Build history of the part. All positions in model axes, mm. Face numbers are marked on the shaded views. A direction names the side the tool comes from. Give positions to 0.01 mm unless a question says otherwise; leave off trailing zeros. Order: outer loops, then holes, each group sorted by start corner. A loop starts at its lowest first (then second) coordinate and runs counter-clockwise, first axis right, second up. Notation, with made-up numbers: M 26,-26.5 L 83,-26.5 A18 ccw 83,0.5 Z; hole C 83,44.25 d3. An arc over 180 degrees is marked long. One line per item, written item: value. Start each with the question number.
from build123d import *

# Parameters (mm, degrees)
SKICA1_W                 = 50
SKICA1_H                 = 65
P_IDAT_VYSUNUT_M1_DEPTH  = 30
P_IDAT_VYSUNUT_M2_DEPTH  = 50
ODEBRAT_VYSUNUT_M1_DEPTH = 18.9
SKICA6_R                 = 2.8
ODEBRAT_VYSUNUT_M2_DEPTH = 58.744783314
SKICA7_R                 = 7.5
ODEBRAT_VYSUNUT_M3_DEPTH = 8.7
SKICA8_R                 = 2.35
ODEBRAT_VYSUNUT_M4_DEPTH = 8.5


with BuildPart() as part:
    # Skica1 → Přidat vysunutím1 (new body)
    with BuildSketch(Plane.XY):
        Rectangle(SKICA1_W, SKICA1_H)
    extrude(amount=P_IDAT_VYSUNUT_M1_DEPTH)

    # Skica3 → Přidat vysunutím2 (add, through all)
    with BuildSketch(Plane(origin=(25, 0, 0), x_dir=(0, 0, -1), z_dir=(1, 0, 0))):
        Polygon((0, 32.5), (0, 48.5), (-30, 32.5), align=None)
    extrude(amount=-P_IDAT_VYSUNUT_M2_DEPTH)

    # Skica5 → Odebrat vysunutím1 (cut)
    with BuildSketch(Plane.XY.offset(30)):
        Polygon((-20.3, 31.35), (20.31, 31.35), (22.6, -31.35), (-22.6, -31.35), align=None)
    extrude(amount=-ODEBRAT_VYSUNUT_M1_DEPTH, mode=Mode.SUBTRACT)

    # Skica6 → Odebrat vysunutím2 (cut, through all)
    with BuildSketch(Plane.XY.offset(11.1)):
        Circle(SKICA6_R)
    extrude(amount=-ODEBRAT_VYSUNUT_M2_DEPTH, mode=Mode.SUBTRACT)

    # Skica7 → Odebrat vysunutím3 (cut)
    with BuildSketch(Plane(origin=(0, 0, 0), x_dir=(-1, 0, 0), z_dir=(0, 0, -1))):
        Circle(SKICA7_R)
    extrude(amount=-ODEBRAT_VYSUNUT_M3_DEPTH, mode=Mode.SUBTRACT)

    # Skica8 → Odebrat vysunutím4 (cut)
    with BuildSketch(Plane(origin=(0, 0, 0), x_dir=(-1, 0, 0), z_dir=(0, 0, -1))):
        with Locations((7.14901322, 26.607213292)):
            Circle(SKICA8_R)
        with Locations(Location((-7.14901322, 26.607213292, 0), (0, 0, 180))):
            Circle(SKICA8_R)
        with Locations(Location((7.14901322, 37.192786708, 0), (0, 0, 180))):
            Circle(SKICA8_R)
        with Locations((-7.14901322, 37.192786708)):
            Circle(SKICA8_R)
    extrude(amount=-ODEBRAT_VYSUNUT_M4_DEPTH, mode=Mode.SUBTRACT)


solid = part.part
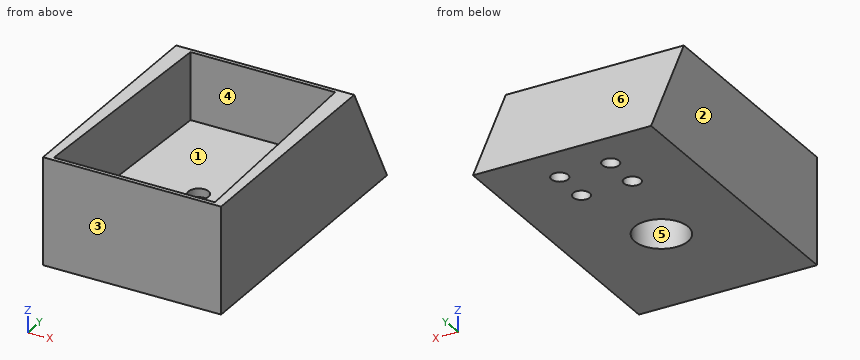
1) Pull direction Y, two halves, no side cores. Call the marked faces 1, 2 and 3: pulls with the +Y half, pulls with the -Y half, needs draft (parallel to the pull), parting line crosses it, or undercut.
2) Tool access for the marked faces 4, 5 and 6: list every direction of +Z, -Z, +X, -X, +Y, -Y with a clear straight run to the whole face (end or side of a thin tool).
3) Slice it at B-B (z = 15). List the corners of the cut face in (x, y), plus the area to 3 significant figures.
4) Drop flat-ended pins along their axis: P1, Ø2.5, axis at x = 7, y = 26, coming from the -Z side; P2, Ø15, axis at x = -6, z = 25, coming from the +Y side; P3, Ø5.5, axis at x = -7.15, y = 37.19, coming from the +Z side. Give the stop position or say it passes through.
5) Slice it at D-D (x = -13.5). List the corners of the cut face in (y, z), plus the area to 3 significant figures.
6) Slice it at C-C (y = 0). List the corners of the cut face in (x, z) (3 decimals), plus the area to 3 significant figures.
7) Drill centre lines: line 1 (X direction, y = 25.5, z = 3.25); line 2 (Z direction, x = 12, y = -28.5); line 3 (Y direction, x = 0, z = 3.25). Where is each one in solid material? Low to high.
8) Slice it at A-A (x = 0). List the corners of the cut face in (y, z).
Results list:
1. face 1: undercut
1. face 2: needs draft
1. face 3: pulls with the -Y half
2. face 4: +Z
2. face 5: -Z
2. face 6: +Z, +X, -X, +Y
3. outline: M -25,-32.5 L 25,-32.5 L 25,40.5 L -25,40.5 Z; hole M -22.6,-31.35 L 22.6,-31.35 L 20.31,31.35 L -20.3,31.35 Z
3. area: 960 mm²
4. P1: stops at z = 8.5
4. P2: stops at y = 39.17
4. P3: stops at z = 26.36
5. outline: M -32.5,0 L 48.5,0 L 32.5,30 L 31.35,30 L 31.35,11.1 L -31.35,11.1 L -31.35,30 L -32.5,30 Z
5. area: 1,000 mm²
6. outline: M -25,0 L -7.5,0 L -7.5,8.7 L -2.8,8.7 L -2.8,11.1 L -21.45,11.1 L -21.45,30 L -25,30 Z; M 2.8,8.7 L 7.5,8.7 L 7.5,0 L 25,0 L 25,30 L 21.455,30 L 21.455,11.1 L 2.8,11.1 Z
6. area: 545 mm²
7. line 1: x = -25 to -9.22, -5.08 to 5.08, 9.22 to 25
7. line 2: z = 0 to 11.1
7. line 3: y = -32.5 to -7.5, 7.5 to 46.77
8. outline: M -32.5,0 L -7.5,0 L -7.5,8.7 L -2.8,8.7 L -2.8,11.1 L -31.35,11.1 L -31.35,30 L -32.5,30 Z; M 2.8,8.7 L 7.5,8.7 L 7.5,0 L 48.5,0 L 32.5,30 L 31.35,30 L 31.35,11.1 L 2.8,11.1 Z
